Could you check a few things on this model? Use its own coordinates, in mm. Give positions to 0.01 mm unless a question says otherwise; leave off trailing zeros. Loops run counter-clockwise (first coordinate to the right, second up) from the corner with the lowest first, then second, coordinate; pieces in that order, holes last. Notation, with made-up numbers: M -23.5,-33 L -3.5,-33 A31 cw -3.5,3 Z; hole C 63.25,-3 d7. An arc over 180 degrees is marked long. Use CSV: the item, a comma, the result in double quotes.
Autodesk Inventor part; units mm, degrees
ref_plane "YZ Plane" through (0, 0, 0) normal (1, 0, 0) x (0, 1, 0)
ref_plane "XZ Plane" through (0, 0, 0) normal (0, 1, 0) x (-1, 0, 0)
ref_plane "XY Plane" through (0, 0, 0) normal (0, 0, 1) x (1, 0, 0)
sketch "Sketch1" plane through (0, 0, 0) normal (0, 1, 0) x (-1, 0, 0)
  line L0 (0, 0) -> (-11.2, 0)
  line L1 (-11.2, 0) -> (-11.2, -25)
  line L2 (-11.2, -25) -> (0, -25)
  line L3 (0, -25) -> (0, 0)
  circle A0 centre (-5.6, -4) radius 2
  circle A1 centre (-5.6, -21) radius 2
  dimension "d0" = 25
  dimension "d1" = 11.2
  dimension "d7" = 4
  dimension "d8" = 4
  dimension "d9" = 17
  dimension "d10" = 5.6
  dimension "d11" = 4
  dimension "d12" = 4
extrude "Extrusion1" add sketch "Sketch1" along normal blind 1
properties part number "Adjustments"
1. I'm going to push a flat-ended pin straight in: pin 1 Ø2.5 at (x, z) = (5.6, -21) entering from +Y. Where does the tip first touch, or does it pass through?
Outcome:
pin 1,"through"
2. I want a section at A-A, the plane z = -21. List the corners of the cut face in (x, y) for me, then the cut area to 3 significant figures.
Outcome:
outline,"M 0,0 L 3.6,0 L 3.6,1 L 0,1 Z; M 7.6,0 L 11.2,0 L 11.2,1 L 7.6,1 Z"
area,"7.20 mm2"
3. Please list where these lines run through material, in increasing order: line 1 (Z direction, x = 5.6, y = 0.65); line 2 (Z direction, x = 7, y = 0.7); line 3 (X direction, y = 0.65, z = -19.75).
Outcome:
line 1,"-25 to -23, -19 to -6, -2 to 0"
line 2,"-25 to -22.43, -19.57 to -5.43, -2.57 to 0"
line 3,"0 to 4.04, 7.16 to 11.2"
4. I want a section at B-B, the plane x = 5.6. List the corners of the cut face in (y, z) for me, then the cut area to 3 significant figures.
Outcome:
outline,"M 0,-25 L 1,-25 L 1,-23 L 0,-23 Z; M 0,-19 L 1,-19 L 1,-6 L 0,-6 Z; M 0,-2 L 1,-2 L 1,0 L 0,0 Z"
area,"17.0 mm2"
5. I want a section at C-C, the plane y = 0.85. List the corners of the cut face in (x, z) for me, then the cut area to 3 significant figures.
Outcome:
outline,"M 0,-25 L 11.2,-25 L 11.2,0 L 0,0 Z; hole C 5.6,-21 d4; hole C 5.6,-4 d4"
area,"255 mm2"
6. If we mould it in two halves opening along Z, with no side actions, what happens to faces 1 (the face through (7.2, 0.5, -2.8)), 2 (the face through (0, 0.5, -12.7)), 3 (the face through (7.074, 0.493, -22.352)), 4 (the face through (5.7, 0.5, -25))? For each: +Z half, -Z half, draft (parallel to the pull), parting line (faces both ways), or undercut.
Outcome:
face 1,"undercut"
face 2,"draft"
face 3,"undercut"
face 4,"-Z half"
